Geometry check sheet. Reference: the model listing, model coordinates, mm. A direction names the side the tool comes from. Give positions to 0.01 mm unless a question says otherwise; leave off trailing zeros. Loops run counter-clockwise (first coordinate to the right, second up) from the corner with the lowest first, then second, coordinate; pieces in that order, holes last. Notation, with made-up numbers: (54.5, -23) -> (101.5, -23) arc R12 ccw to (101.5, -2) -> close; hole circle Ø8 at (88.25, 15). An arc over 180 degrees is marked (long way). One line per question, with ' | ' between items.
from build123d import *

# Parameters (mm, degrees)
F0_R      = 5
F1_DEPTH  = 8
F2_R      = 3
F3_DEPTH  = 42
F4_R      = 12
F5_DEPTH  = 12
F6_W      = 20
F6_H      = 20
F7_DEPTH  = 10
F10_DEPTH = 2


with BuildPart() as f1:
    # F0 (on Front) → F1 (new body)
    with BuildSketch(Plane.XZ):
        Circle(F0_R)
    extrude(amount=F1_DEPTH)

    # F2 (on face) → F3 (join)
    with BuildSketch(Plane.XZ.offset(8)):
        Circle(F2_R)
    extrude(amount=F3_DEPTH)

    # F4 (on Front) → F5 (join)
    with BuildSketch(Plane.XZ):
        Circle(F4_R)
    extrude(amount=-F5_DEPTH)

    # F6 (on face) → F7 (join)
    with BuildSketch(Plane(origin=(0, 12, 0), x_dir=(-1, 0, 0), z_dir=(0, 1, 0))):
        with Locations((0, -10)):
            Rectangle(F6_W, F6_H)
    extrude(amount=-F7_DEPTH)

    # F9 (on offset) → F10 (join)
    with BuildSketch(Plane.XZ.offset(6)):
        Polygon((7, -4.041452), (7, 4.041452), (0, 8.082904), (-7, 4.041452), (-7, -4.041452), (0, -8.082904), align=None)
    extrude(amount=-F10_DEPTH)


solid = f1.part
Item 1: Sectioned sample at A-A (z = 0). Record the cut outline in (x, y).
Result:
outline: (-12, 0) -> (-5, 0) -> (-5, -4) -> (-7, -4) -> (-7, -6) -> (-5, -6) -> (-5, -8) -> (-3, -8) -> (-3, -50) -> (3, -50) -> (3, -8) -> (5, -8) -> (5, -6) -> (7, -6) -> (7, -4) -> (5, -4) -> (5, 0) -> (12, 0) -> (12, 12) -> (-12, 12) -> close
Item 2: Sectioned sample at C-C (z = -17). Record the cut outline in (x, y), plus the area to 3 significant figures.
Result:
outline: (-10, 2) -> (10, 2) -> (10, 12) -> (-10, 12) -> close | area: 200 mm2
Item 3: Scan lines: probe 1 along Y at (x, z) = (4.75, -4); probe 2 along Y at (x, z) = (8, -3.5); probe 3 along X at (y, z) = (8.5, -11). Record each from-to range of solid material in increasing order.
Result:
probe 1: -6 to -4, 0 to 12 | probe 2: 0 to 12 | probe 3: -10 to 10
Item 4: Release check for a two-part mould opening along Y. For faces 1 (the face through (-5, -4, -2)), 2 (the face through (7, -5, 0)), 3 (the face through (5.2, 0, 0.2)), 4 (the face through (0, 2, -15)) record: pulls with the +Y half, pulls with the -Y half, needs draft (parallel to the pull), parting line crosses it, or undercut.
Result:
face 1: undercut | face 2: needs draft | face 3: undercut | face 4: pulls with the -Y half
Item 5: Sectioned sample at D-D (y = -31). Record the cut outline in (x, z).
Result:
outline: circle Ø6 at (0, 0)
Item 6: Depth check by flat-ended pin: pin 1 Ø0.6 at (y, z) = (-5, -0.5) entering from -X; pin 2 Ø8 at (x, y) = (1, -9) entering from +Z; pin 3 Ø11 at (y, z) = (7, -11.5) entering from -X. Enter the tip coordinate at first touch or a pass-through.
Result:
pin 1: x = -7 | pin 2: z = 8.08 | pin 3: x = -10.39
Item 7: Set-up check for faces 5 (the face through (-7, -5, 0)), 6 (the face through (3.549, -5.014, 6.034)), 7 (the face through (-3.549, -5.014, -6.034)): record each of +Z, -Z, +X, -X, +Y, -Y from which the full face is reachable in a straight line by a thin tool's end or side.
Result:
face 5: +Z, -Z, -X, -Y | face 6: +Z, +X, -Y | face 7: -Z, -X, -Y
Item 8: Sectioned sample at B-B (y = -5). Record the cut outline in (x, z), plus the area to 3 significant figures.
Result:
outline: (-7, -4.04) -> (0, -8.08) -> (7, -4.04) -> (7, 4.04) -> (0, 8.08) -> (-7, 4.04) -> close | area: 170 mm2
